from build123d import *

# Parameters (mm, degrees)
BOSS_EXTRUDE1_DEPTH = 7
BOSS_EXTRUDE2_DEPTH = 20
SKETCH3_R           = 2.25
CUT_EXTRUDE1_DEPTH  = 8
SKETCH4_R           = 2.25
CUT_EXTRUDE2_DEPTH  = 8
SKETCH5_R           = 1.85
CUT_EXTRUDE4_DEPTH  = 3
SKETCH6_R           = 1.85
CUT_EXTRUDE5_DEPTH  = 3
SKETCH7_R           = 1.85
CUT_EXTRUDE6_DEPTH  = 3


with BuildPart() as part:
    # Sketch1 → Boss-Extrude1 (new body)
    with BuildSketch(Plane(origin=(0, 0, 0), x_dir=(1, 0, 0), z_dir=(0, 1, 0))):
        Polygon((12.092522712, -8.5), (30, -8.5), (30, 8.5), (12.092522712, 8.5), (8.5, 14.722431864), (8.5, 32), (-8.5, 32), (-8.5, 14.722431864), (-12.092522712, 8.5), (-30, 8.5), (-30, -8.5), (-12.092522712, -8.5), (-8.5, -14.722431864), (-8.5, -32), (8.5, -32), (8.5, -14.722431864), align=None)
        Polygon((-11.547005384, 0), (-5.773502692, 10), (5.773502692, 10), (11.547005384, 0), (5.773502692, -10), (-5.773502692, -10), align=None, mode=Mode.SUBTRACT)
    extrude(amount=BOSS_EXTRUDE1_DEPTH)

    # Sketch2 → Boss-Extrude2 (add)
    with BuildSketch(Plane(origin=(0, 7, 0), x_dir=(1, 0, 0), z_dir=(0, 1, 0))):
        Polygon((-15.011106999, 0), (-7.505553499, -13), (7.505553499, -13), (15.011106999, 0), (7.505553499, 13), (-7.505553499, 13), align=None)
        Polygon((-11.547005384, 0), (-5.773502692, -10), (5.773502692, -10), (11.547005384, 0), (5.773502692, 10), (-5.773502692, 10), align=None, mode=Mode.SUBTRACT)
    extrude(amount=BOSS_EXTRUDE2_DEPTH)

    # Sketch3 → Cut-Extrude1 (cut, through all)
    with BuildSketch(Plane(origin=(0, 7, 0), x_dir=(1, 0, 0), z_dir=(0, 1, 0))):
        with Locations(Location((0, 25, 0), (0, 0, 270))):  # turned: the seam where the file's is
            Circle(SKETCH3_R)
    cut_extrude1 = extrude(amount=-CUT_EXTRUDE1_DEPTH, mode=Mode.SUBTRACT)

    # Mirror1: Cut-Extrude1 across plane
    add(cut_extrude1.mirror(Plane.XY), mode=Mode.SUBTRACT)

    # Sketch4 → Cut-Extrude2 (cut, through all)
    with BuildSketch(Plane(origin=(0, 7, 0), x_dir=(1, 0, 0), z_dir=(0, 1, 0))):
        with Locations(Location((-24, 0, 0), (0, 0, 270))):  # turned: the seam where the file's is
            Circle(SKETCH4_R)
    cut_extrude2 = extrude(amount=-CUT_EXTRUDE2_DEPTH, mode=Mode.SUBTRACT)

    # Mirror2: Cut-Extrude2 across plane
    add(cut_extrude2.mirror(Plane(origin=(0, 0, 0), x_dir=(0, 0, 1), z_dir=(1, 0, 0))), mode=Mode.SUBTRACT)

    # Sketch5 → Cut-Extrude4 (cut)
    with BuildSketch(Plane.XY.offset(13)):
        with Locations((0, 17)):
            Circle(SKETCH5_R)
    extrude(amount=-CUT_EXTRUDE4_DEPTH, mode=Mode.SUBTRACT)

    # Sketch6 → Cut-Extrude5 (cut)
    with BuildSketch(Plane(origin=(11.258330249, 0, -6.5), x_dir=(-0.5, 0, -0.866025404), z_dir=(0.866025404, 0, -0.5))):
        with Locations((0, 17)):
            Circle(SKETCH6_R)
    extrude(amount=-CUT_EXTRUDE5_DEPTH, mode=Mode.SUBTRACT)

    # Sketch7 → Cut-Extrude6 (cut)
    with BuildSketch(Plane(origin=(-11.258330249, 0, -6.5), x_dir=(-0.5, 0, 0.866025404), z_dir=(-0.866025404, 0, -0.5))):
        with Locations((0, 17)):
            Circle(SKETCH7_R)
    extrude(amount=-CUT_EXTRUDE6_DEPTH, mode=Mode.SUBTRACT)


solid = part.part
Work out the finished part from the listing and answer in its coordinate system (mm). A direction names the side the tool comes from. Round coordinates to 2 decimals unless told otherwise and drop trailing zeros. Write each loop counter-clockwise with the first axis right and the second up, starting at its lowest first coordinate (ties: lowest second). Pieces come first, ordered by that corner, then holes.
1) A cutting plane is placed at A-A (x = 0). Give the vertices of the cut face in (y, z), plus the area to 3 significant figures.
2) Straight lines are drawn through the part: line 1 (X direction, y = 2, z = 0); line 2 (Z direction, x = 24, y = 2.5); line 3 (Z direction, x = 0, y = 14). For each, find the intervals that lie inside material, in ascending order.
3) A cutting plane is placed at C-C (z = -25). Give the vertices of the cut face in (x, y), plus the area to 3 significant figures.
4) A cutting plane is placed at B-B (y = 2.25). Give the vertices of the cut face in (x, z), plus the area to 3 significant figures.
5) Given pin 1 Ø7.5 at (x, y) = (22, 2.5) entering from -Z; pin 2 Ø3.5 at (y, z) = (2, -20) entering from +X; pin 3 Ø4 at (y, z) = (17, 6.5) entering from -X; pin 4 Ø10 at (y, z) = (19, 21.5) entering from -X, each flat-ended and moving along its own axis, determine where each tip first touches the part or whether it passes through.
6) The mould has two halves that part along X. Classify faces 5 (the flat face through (11.2, 16.9, 6.6)), 6 (the flat face through (0, 7, -15)), 7 (the flat face through (0, 13, 10)): pulls with the +X half, pulls with the -X half, needs draft (parallel to the pull), parting line crosses it, or undercut.
7) A cutting plane is placed at D-D (x = -24). Give the vertices of the cut face in (y, z).
8) A tool of negligible diameter and unlimited length cuts with its end or side. For faces 1 (the flat face through (-11.31, 16.86, 6.41)), 2 (the flat face through (-21, 3, -8.5)), 3 (the flat face through (8.62, 13.31, 5.07)), 4 (the flat face through (11.31, 14.64, -6.41)), from which of +Z, -Z, +X, -X, +Y, -Y can it reach the whole face along a straight path? Write none if from no direction.
Completed:
1. outline: (0, -32) - (7, -32) - (7, -27.25) - (0, -27.25) - close; (0, -22.75) - (7, -22.75) - (7, -13) - (27, -13) - (27, -10) - (0, -10) - close; (0, 10) - (15.15, 10) - (15.15, 13) - (7, 13) - (7, 22.75) - (0, 22.75) - close; (0, 27.25) - (7, 27.25) - (7, 32) - (0, 32) - close; (18.85, 10) - (27, 10) - (27, 13) - (18.85, 13) - close
1. area: 354 mm2
2. line 1: x = -30 to -26.25, -21.75 to -11.55, 11.55 to 21.75, 26.25 to 30
2. line 2: z = -8.5 to -2.25, 2.25 to 8.5
2. line 3: z = -13 to -10, 10 to 13
3. outline: (-8.5, 0) - (-2.25, 0) - (-2.25, 7) - (-8.5, 7) - close; (2.25, 0) - (8.5, 0) - (8.5, 7) - (2.25, 7) - close
3. area: 87.5 mm2
4. outline: (-30, -8.5) - (-12.09, -8.5) - (-8.5, -14.72) - (-8.5, -32) - (8.5, -32) - (8.5, -14.72) - (12.09, -8.5) - (30, -8.5) - (30, 8.5) - (12.09, 8.5) - (8.5, 14.72) - (8.5, 32) - (-8.5, 32) - (-8.5, 14.72) - (-12.09, 8.5) - (-30, 8.5) - close; hole circle Ø4.5 at (-24, 0); hole (-11.55, 0) - (-5.77, -10) - (5.77, -10) - (11.55, 0) - (5.77, 10) - (-5.77, 10) - close; hole circle Ø4.5 at (0, -25); hole circle Ø4.5 at (0, 25); hole circle Ø4.5 at (24, 0)
4. area: 1,450 mm2
5. pin 1: stops at z = -8.5
5. pin 2: stops at x = 8.5
5. pin 3: stops at x = -12.41
5. pin 4: passes through
6. face 5: pulls with the +X half
6. face 6: needs draft
6. face 7: undercut
7. outline: (0, -8.5) - (7, -8.5) - (7, -2.25) - (0, -2.25) - close; (0, 2.25) - (7, 2.25) - (7, 8.5) - (0, 8.5) - close
8. face 1: +Z, -X, +Y
8. face 2: -Z, -X, +Y, -Y
8. face 3: +Y, -Y
8. face 4: -Z, +X, +Y
